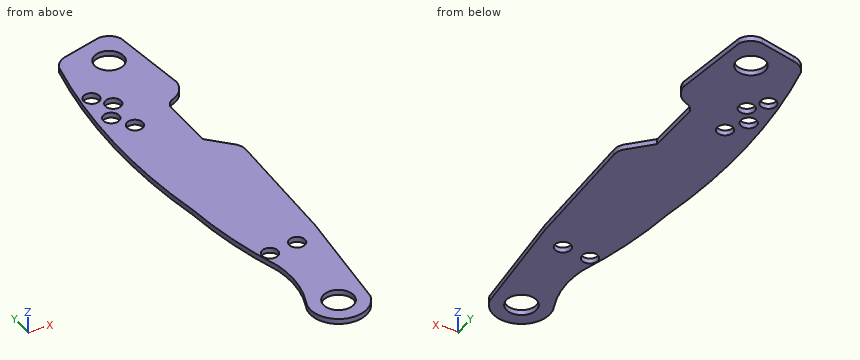
from build123d import *

# Parameters (mm, degrees)
SKETCH1_R           = 2.159
SKETCH1_R_2         = 1.143
SKETCH1_R_3         = 2.0955
BOSS_EXTRUDE1_DEPTH = 0.381


with BuildPart() as part:
    # Sketch1 → Boss-Extrude1 (new body, symmetric)
    with BuildSketch(Plane.XY):
        with BuildLine():
            Line((74.009533162, 2.524763773), (72.281998937, -13.985236227))
            ThreePointArc((72.281998937, -13.985236227), (66.894838719, -16.481573981), (64.766369935, -10.938757185))
            ThreePointArc((64.766369935, -10.938757185), (65.80913713, -6.8614285), (65.635785401, -2.656440771))
            ThreePointArc((65.635785401, -2.656440771), (63.616027596, 5.10567878), (62.526786778, 13.051965708))
            ThreePointArc((62.526786778, 13.051965708), (61.351286871, 30.387313841), (63.589596905, 47.617695819))
            ThreePointArc((63.589596905, 47.617695819), (64.412502938, 48.666218898), (65.627533162, 49.214193845))
            Line((65.627533162, 49.214193845), (70.834533162, 50.498790171))
            ThreePointArc((70.834533162, 50.498790171), (72.374643438, 50.21510876), (73.370794631, 49.006763773))
            Line((73.370794631, 49.006763773), (74.635112814, 37.576763773))
            ThreePointArc((74.635112814, 37.576763773), (73.946841775, 35.757603322), (72.379792613, 34.605466744))
            ThreePointArc((72.379792613, 34.605466744), (71.641962058, 34.084204846), (71.274872248, 33.258763773))
            Line((71.274872248, 33.258763773), (71.274872248, 25.384763773))
            Line((71.274872248, 25.384763773), (73.922374141, 22.590763773))
            ThreePointArc((73.922374141, 22.590763773), (74.599970213, 21.681643486), (74.757378227, 20.558763773))
            Line((74.757378227, 20.558763773), (74.009533162, 2.524763773))
        make_face()
        with Locations((68.421533162, -12.715236227)):
            Circle(SKETCH1_R, mode=Mode.SUBTRACT)
        with Locations((70.224933162, 0.492763773)):
            Circle(SKETCH1_R_2, mode=Mode.SUBTRACT)
        with Locations((66.135533162, 0.202809344)):
            Circle(SKETCH1_R_2, mode=Mode.SUBTRACT)
        with Locations((65.500533162, 32.242763773)):
            Circle(SKETCH1_R_2, mode=Mode.SUBTRACT)
        with Locations((65.500533162, 37.576763773)):
            Circle(SKETCH1_R_2, mode=Mode.SUBTRACT)
        with Locations((69.691533162, 45.704763773)):
            Circle(SKETCH1_R_3, mode=Mode.SUBTRACT)
        with Locations((63.722533162, 39.862763773)):
            Circle(SKETCH1_R_2, mode=Mode.SUBTRACT)
        with Locations((63.722533162, 35.036763773)):
            Circle(SKETCH1_R_2, mode=Mode.SUBTRACT)
    extrude(amount=BOSS_EXTRUDE1_DEPTH, both=True)


solid = part.part
Verification items for the finished model (mm, model axes). Round coordinates to 2 decimals unless told otherwise and drop trailing zeros. Order: outer loops, then holes, each group sorted by start corner. A loop starts at its lowest first (then second) coordinate and runs counter-clockwise, first axis right, second up.
1. Thickness scan on L1, parallel to Y at x = 67, z = -0.1; L2, parallel to X at y = 0, z = 0.1; L3, parallel to Y at x = 69.25, z = 0.1. Record the ranges inside material, lowest first.
Final values:
L1: y = -16.52 to -14.34, -11.09 to -0.54, 0.95 to 49.55
L2: x = 64.83 to 65.01, 67.26 to 69.19, 71.26 to 73.75
L3: y = -16.69 to -14.71, -10.72 to -0.1, 1.09 to 43.66, 47.75 to 50.11
2. Section check B-B on y = 11. Record the cut outline in (x, z).
Final values:
outline: (62.72, -0.38) - (74.36, -0.38) - (74.36, 0.38) - (62.72, 0.38) - close
3. Section check A-A on z = 0.25. State how many separate pieces and enclosed holes the cut face has, then the cut area to 3 significant figures.
Final values:
separate pieces: 1
enclosed holes: 8
area: 626 mm2
4. Go/stop test with a flat-tipped pin: P1, Ø3, axis at x = 63.72, y = 35.04, coming from the +Z side. Record where the tip stops, or that it passes through.
Final values:
P1: stops at z = 0.38
5. Section check C-C on y = 29.5. Record the cut outline in (x, z), then the cut area to 3 significant figures.
Final values:
outline: (61.33, -0.38) - (71.27, -0.38) - (71.27, 0.38) - (61.33, 0.38) - close
area: 7.58 mm2
